Can you work these out from the model? Positions are in its coordinate system, mm. A direction names the side the tool comes from. Coordinates: 2 decimals unless noted, no trailing zeros. Loops run counter-clockwise (first coordinate to the right, second up) from the corner with the lowest first, then second, coordinate; pieces in that order, holes last. Notation, with made-up numbers: (73.5, -8) -> (115.5, -8) arc R26 cw to (115.5, 17) -> close; hole circle Ø2 at (0.25, 44.5). An arc over 180 degrees is marked (long way). Put each result on its own line as item: value. Start each with the question number.
Item 1: If we section it at C-C on z = -0.5: Please give me the cut outline in (x, y).
Item 2: Please list where these lines run through material, in increasing order: L1, parallel to Y at x = 0.1, z = 1; L2, parallel to Z at x = 1.45, y = 1.4; L3, parallel to X at y = 0.7, z = -2.5. Write a range as from..to.
Item 3: We'd pull the mould along Y, two halves only. Please class faces 3 (the flat face through (0, 0, 1.2)), 4 (the cylindrical face through (1, 0.32, -3.45)), 5 (the flat face through (-1, 1, 0)): pulls with the +Y half, pulls with the -Y half, needs draft (parallel to the pull), parting line crosses it, or undercut.
Item 4: If we section it at A-A on x = 0: Please give me the cut outline in (y, z) (3 decimals).
Item 5: Will these pins go through, and if not, where does the flat tip stop? P1, Ø0.6, axis at y = 0, z = 1.5, coming from the +X side; P2, Ø1.5, axis at x = 1.5, z = -3, coming from the +Y side; P3, Ø0.6, axis at y = 0, z = 1.5, coming from the -X side.
Item 6: For faces 1 (the cylindrical face through (1.29, 2.024, 0.304)), 2 (the cylindrical face through (-0.224, 1.705, 1.006)), which set-ups out of +Z, -Z, +X, -X, +Y, -Y let a thin tool reach every point of the face, with its end or its side?
Item 7: If we section it at D-D on z = 0.75: Please give me the cut outline in (x, y), plus the area to 3 significant figures.
```python
from build123d import *

# Parameters (mm, degrees)
POCKET_DEPTH = 0.5
FILLET_R     = 0.3


with BuildPart() as part:
    # Sketch001 → Revolution (revolve)
    with BuildSketch(Plane.XZ):
        Polygon((1.05, -7), (1.05, 0), (2.4, 0), (2.4, 0.6), (1.72, 0.6), (1.72, 1.7), (0, 1.7), (0, -7), align=None)
    revolve(axis=Axis((0, 0, 0), (0, 0, 1)))

    # Sketch → Pocket (cut)
    with BuildSketch(Plane(origin=(0, 0, 1.7), x_dir=(-1, 0, 0), z_dir=(0, 0, 1))):
        Polygon((-0.25, 0.875), (0.25, 0.875), (0.25, 0.25), (0.875, 0.25), (0.875, -0.25), (0.25, -0.25), (0.25, -0.875), (-0.25, -0.875), (-0.25, -0.25), (-0.875, -0.25), (-0.875, 0.25), (-0.25, 0.25), align=None)
    extrude(amount=-POCKET_DEPTH, mode=Mode.SUBTRACT)

    # Fillet
    fillet_edges = [part.edges().sort_by_distance(p)[0] for p in [
        (-1.72, 0, 1.7),
    ]]
    fillet(fillet_edges, radius=FILLET_R)


solid = part.part
```
Solutions:
1. outline: circle Ø2.1 at (0, 0)
2. L1: -1.72..1.72
2. L2: 0..0.6
2. L3: -0.78..0.78
3. face 3: undercut
3. face 4: parting line crosses it
3. face 5: needs draft
4. outline: (-2.4, 0) -> (-1.05, 0) -> (-1.05, -7) -> (1.05, -7) -> (1.05, 0) -> (2.4, 0) -> (2.4, 0.6) -> (1.72, 0.6) -> (1.72, 1.4) arc R0.3 ccw to (1.42, 1.7) -> (0.875, 1.7) -> (0.875, 1.2) -> (-0.875, 1.2) -> (-0.875, 1.7) -> (-1.42, 1.7) arc R0.3 ccw to (-1.72, 1.4) -> (-1.72, 0.6) -> (-2.4, 0.6) -> close
5. P1: x = 1.72
5. P2: y = 0.73
5. P3: x = -1.72
6. face 1: +Z, -Z
6. face 2: +Z
7. outline: circle Ø3.44 at (0, 0)
7. area: 9.29 mm^2
